from build123d import *

# Parameters (mm, degrees)
SKETCH1_R               = 2.3622
BASE_EXTRUDE_DEPTH      = 1.651
SKETCH3_R               = 2.921
BOSS_EXTRUDE1_DEPTH     = 0.762
SKETCH4_R               = 2.3876
BOSS_EXTRUDE2_DEPTH     = 7.239
SKETCH7_R               = 1.4605
CUT_EXTRUDE2_DEPTH      = 11.498837364
CUT_EXTRUDE4_DEPTH      = 10.004470257
CUT_EXTRUDE4_DEPTH_BACK = 10.004470257
BOSS_EXTRUDE11_START    = -3.937
BOSS_EXTRUDE11_DEPTH    = 3.937
CIRPATTERN1_COUNT       = 4


with BuildPart() as part:
    # Sketch1 → Base-Extrude (new body)
    with BuildSketch(Plane(origin=(0, 0, 0), x_dir=(0, 0, -1), z_dir=(1, 0, 0))):
        with Locations(Location((0, 0, 0), (0, 0, 180))):
            Circle(SKETCH1_R)
    extrude(amount=BASE_EXTRUDE_DEPTH)

    # Sketch3 → Boss-Extrude1 (add)
    with BuildSketch(Plane.ZY):
        with Locations(Location((0, 0, 0), (0, 0, 180))):
            Circle(SKETCH3_R)
    extrude(amount=BOSS_EXTRUDE1_DEPTH)

    # Sketch4 → Boss-Extrude2 (add)
    with BuildSketch(Plane.ZY.offset(0.762)):
        Circle(SKETCH4_R)
    extrude(amount=BOSS_EXTRUDE2_DEPTH)

    # Sketch6 → Boss-Revolve2 (revolve)
    with BuildSketch(Plane(origin=(0, 0, 0), x_dir=(1, 0, 0), z_dir=(0, 1, 0)), mode=Mode.PRIVATE) as boss_revolve2_sk:
        with BuildLine():
            Line((-8.001, 2.3876), (-7.112, 2.3876))
            ThreePointArc((-7.112, 2.3876), (-7.5565, 2.54), (-8.001, 2.3876))
        make_face()
    revolve(boss_revolve2_sk.sketch.rotate(Axis((0, 0, 0), (-1, 0, 0)), 180), axis=Axis((0, 0, 0), (-1, 0, 0)))

    # Sketch7 → Cut-Extrude2 (cut, through all)
    with BuildSketch(Plane.ZY.offset(8.001)):
        Circle(SKETCH7_R)
    extrude(amount=-CUT_EXTRUDE2_DEPTH, mode=Mode.SUBTRACT)

    # Sketch8 → Cut-Extrude4 (cut, two sides: drawn at the far end of the back side and taken through both)
    with BuildSketch(Plane(origin=(0, 0, 0), x_dir=(1, 0, 0), z_dir=(0, 1, 0)).offset(-CUT_EXTRUDE4_DEPTH_BACK)):
        with BuildLine():
            Line((-8.001, 0.508), (-5.207, 0.508))
            ThreePointArc((-5.207, 0.508), (-4.699, 0), (-5.207, -0.508))
            Line((-5.207, -0.508), (-8.001, -0.508))
            Line((-8.001, -0.508), (-8.001, 0.508))
        make_face()
    extrude(amount=CUT_EXTRUDE4_DEPTH + CUT_EXTRUDE4_DEPTH_BACK, mode=Mode.SUBTRACT)

    # Sketch11 → Boss-Extrude11 (add)
    with BuildSketch(Plane(origin=(1.651, 0, 0), x_dir=(0, 0, -1), z_dir=(1, 0, 0)).offset(BOSS_EXTRUDE11_START)):
        with BuildLine():
            ThreePointArc((0.39848324, 1.405087669), (0, 1.4605), (-0.39848324, 1.405087669))
            ThreePointArc((-0.39848324, 1.405087669), (0, 1.3716), (0.39848324, 1.405087669))
        make_face()
    boss_extrude11 = extrude(amount=BOSS_EXTRUDE11_DEPTH)

    # CirPattern1: Boss-Extrude11 ×4 about axis
    cirpattern1_axis = Axis((0, 0, 0), (1, 0, 0))
    for i in range(1, CIRPATTERN1_COUNT):
        add(boss_extrude11.rotate(cirpattern1_axis, i * 360 / CIRPATTERN1_COUNT))


solid = part.part
Read the model definition and answer for the solid it produces. Units are mm, in the model's axes. A direction names the side the tool comes from. Round coordinates to 2 decimals unless told otherwise and drop trailing zeros. Order: outer loops, then holes, each group sorted by start corner. A loop starts at its lowest first (then second) coordinate and runs counter-clockwise, first axis right, second up.
1) The part is cut by section B-B on x = 0.75. Write down the section's boundary in (y, z), plus the area to 3 significant figures.
2) Flat-ended cylindrical pins translate along their axes: pin 1 (2.5 mm diameter, centred on y = 0, z = 0, fed in from -X); pin 2 (1.2 mm diameter, centred on x = -7, y = 1.5, fed in from +Z); pin 3 (0.9 mm diameter, centred on x = -6.5, y = -2, fed in from -Z); pin 4 (1.5 mm diameter, centred on x = 0.5, z = -1, fed in from +Y). Find the tip coordinate at first contact, or state that the pin passes through.
3) Straight lines are drawn through the part: L1, parallel to Z at x = -2.75, y = 0; L2, parallel to Z at x = 1.25, y = -0.1. For each, find the intervals that lie inside material, in ascending order.
4) The part is cut by section D-D on x = -5. Write down the section's boundary in (y, z), plus the area to 3 significant figures.
5) The mould has two halves that part along Z. Classify faces 1 (the face through (-3.24, -0.56, 1.35)), 2 (the face through (-8.001, 0, -2)), 3 (the face through (0.81, -1.99, 1.27)), 4 (the face through (-7, 2, 0.508)): released by +Z, released by -Z, zero draft, split by the parting line, or undercut.
6) The part is cut by section A-A on y = 0. Write down the section's boundary in (x, z), plus the area to 3 significant figures.
7) The part is cut by section C-C on z = 0. Write down the section's boundary in (x, y), plus the area to 3 significant figures.
8) For faces 5 (the face through (-7, -2, -0.508)), 6 (the face through (-8.001, 0, 2)), 7 (the face through (-3.89, -2.33, -0.52)), determine the directions among +Z, -Z, +X, -X, +Y, -Y from which every point of the face is accessible in a straight line to the end or side of a thin tool.
Resolved:
1. outline: circle Ø4.72 at (0, 0); hole (-1.41, -0.4) arc R1.46 ccw to (-0.4, -1.41) arc R2.39 cw to (0.4, -1.41) arc R1.46 ccw to (1.41, -0.4) arc R2.39 cw to (1.41, 0.4) arc R1.46 ccw to (0.4, 1.41) arc R2.39 cw to (-0.4, 1.41) arc R1.46 ccw to (-1.41, 0.4) arc R2.39 cw to start
1. area: 11.0 mm2
2. pin 1: passes through
2. pin 2: stops at z = 2.3
2. pin 3: stops at z = -1.82
2. pin 4: stops at y = 2.89
3. L1: z = -2.39 to -1.46, 1.46 to 2.39
3. L2: z = -2.36 to -1.37, 1.37 to 2.36
4. outline: (-2.34, -0.46) arc R2.39 ccw to (2.34, -0.46) - (1.38, -0.46) arc R1.46 cw to (-1.38, -0.46) - close; (-2.34, 0.46) - (-1.38, 0.46) arc R1.46 cw to (1.38, 0.46) - (2.34, 0.46) arc R2.39 ccw to start
4. area: 9.47 mm2
5. face 1: undercut
5. face 2: zero draft
5. face 3: split by the parting line
5. face 4: undercut
6. outline: (-8, -2.39) arc R0.72 ccw to (-7.11, -2.39) - (-0.76, -2.39) - (-0.76, -2.92) - (0, -2.92) - (0, -2.36) - (1.65, -2.36) - (1.65, -1.37) - (-2.29, -1.37) - (-2.29, -1.46) - (-8, -1.46) - close; (-8, 1.46) - (-2.29, 1.46) - (-2.29, 1.37) - (1.65, 1.37) - (1.65, 2.36) - (0, 2.36) - (0, 2.92) - (-0.76, 2.92) - (-0.76, 2.39) - (-7.11, 2.39) arc R0.72 ccw to (-8, 2.39) - close
6. area: 19.5 mm2
7. outline: (-4.7, -2.39) - (-0.76, -2.39) - (-0.76, -2.92) - (0, -2.92) - (0, -2.36) - (1.65, -2.36) - (1.65, -1.37) - (-2.29, -1.37) - (-2.29, -1.46) - (-4.7, -1.46) - close; (-4.7, 1.46) - (-2.29, 1.46) - (-2.29, 1.37) - (1.65, 1.37) - (1.65, 2.36) - (0, 2.36) - (0, 2.92) - (-0.76, 2.92) - (-0.76, 2.39) - (-4.7, 2.39) - close
7. area: 13.2 mm2
8. face 5: -X, +Y, -Y
8. face 6: +Z, -Z, -X, +Y, -Y
8. face 7: none
